Geometry: see drawing. Coordinates: mm, zero at the bounding-box minimum. A direction names the side the tool comes from. Give positions to 0.01 mm unless a question says otherwise; leave off trailing zeros. Write each loop counter-clockwise with the first axis right and the second up, starting at its lowest first coordinate (ties: lowest second). Pieces come first, ordered by that corner, then holes. Notation, with made-up numbers: (-15, -22.75) - (28, -22.75) arc R26 cw to (28, 12.25) - close; hole circle Ø4 at (47, -8.5). An arc over 180 degrees is marked (long way). Use CSV: the item, a comma, the result in double quotes. Start each with the question number.
(1) Section D-D on z = 1.75. Output: boundary loops of the cut face in (x, y).
(2) Section C-C on z = 0.5. Output: boundary loops of the cut face in (x, y), and give its area (3 significant figures).
(3) Reachability of the marked faces 1 and 2 from +Z, -Z, +X, -X, +Y, -Y: full face, straight path, thin tool, end or side. Return the list, or none.
(4) Draft query along Y for the marked faces 3, 4 and 5. Return one class per face: released by +Y, released by -Y, zero draft, split by the parting line, or undercut.
(5) Section A-A on x = 6.5. Output: boundary loops of the cut face in (y, z), and give its area (3 significant figures).
(6) Line query: probe 1 along X at (y, z) = (5, 3.5); probe 2 along Y at (x, z) = (5.5, 0.6); probe 3 along Z at (x, y) = (9.5, 12). Output: solid intervals per line, ascending. Write a range as [from, to].
(7) First-contact query: pin 1 Ø1.5 at (x, z) = (10, 3) entering from +Y; pin 2 Ø3 at (y, z) = (7.5, 1) entering from -X; pin 3 Ø2 at (x, z) = (5, 4) entering from +Y; pin 4 Ø3 at (x, z) = (8, 3.5) entering from -Y. Flat tips, straight axial feed; report the tip coordinate or a pass-through.
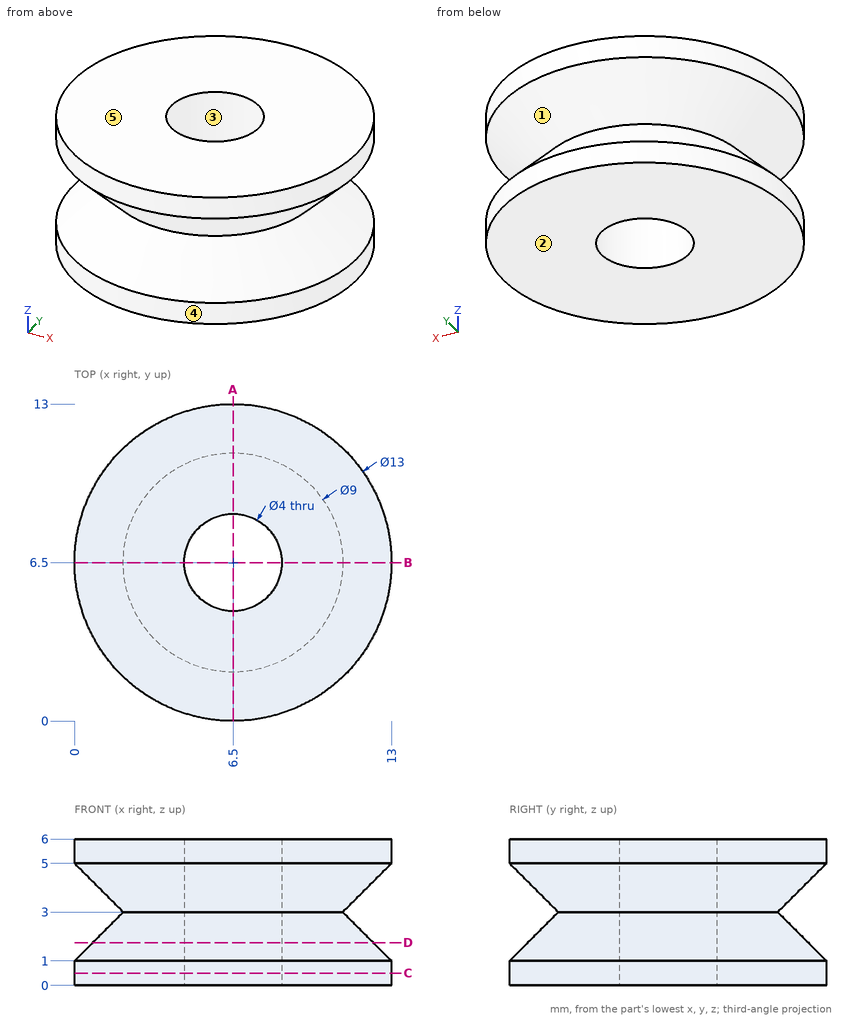
Check values:
1,outline,"circle Ø11.5 at (6.5, 6.5); hole circle Ø4 at (6.5, 6.5)"
2,outline,"circle Ø13 at (6.5, 6.5); hole circle Ø4 at (6.5, 6.5)"
2,area,"120 mm²"
3,face 1,"none"
3,face 2,"-Z, +X, -X, +Y, -Y"
4,face 3,"undercut"
4,face 4,"split by the parting line"
4,face 5,"zero draft"
5,outline,"(0, 0) - (4.5, 0) - (4.5, 6) - (0, 6) - (0, 5) - (2, 3) - (0, 1) - close; (8.5, 0) - (13, 0) - (13, 1) - (11, 3) - (13, 5) - (13, 6) - (8.5, 6) - close"
5,area,"46.0 mm²"
6,probe 1,"x = [1.73, 5.18], [7.82, 11.27]"
6,probe 2,"y = [0.08, 4.77], [8.23, 12.92]"
6,probe 3,"z = [0, 1.24], [4.76, 6]"
7,pin 1,"stops at y = 10.59"
7,pin 2,"stops at x = 0"
7,pin 3,"stops at y = 12.85"
7,pin 4,"stops at y = 0.14"
